Read the model definition and answer for the solid it produces. Units are mm, in the model's axes. Face numbers are marked on the shaded views. A direction names the side the tool comes from. Give positions to 0.01 mm unless a question says otherwise; leave off trailing zeros. Order: outer loops, then holes, each group sorted by start corner. A loop starts at its lowest first (then second) coordinate and runs counter-clockwise, first axis right, second up. Notation, with made-up numbers: (32, 0.5) -> (41, 0.5) arc R7 cw to (41, 9.5) -> close; hole circle Ø9 at (-20.75, 45.5). An arc over 180 degrees is marked (long way). Use one line per item in the form item = value.
```python
from build123d import *

# Parameters (mm, degrees)
F0_W     = 28
F0_H     = 30
F0_W_2   = 20
F0_H_2   = 22
F1_DEPTH = 10
F2_DEPTH = 15
F3_W     = 10
F3_H     = 10
F4_DEPTH = 5


with BuildPart() as f1:
    # F0 (on Top) → F1 (new body)
    with BuildSketch(Plane.XY):
        Rectangle(F0_W, F0_H)
        Rectangle(F0_W_2, F0_H_2, mode=Mode.SUBTRACT)
    extrude(amount=F1_DEPTH)

    # F0 (on Top) → F2 (join)
    with BuildSketch(Plane.XY):
        Rectangle(F0_W_2, F0_H_2)
    extrude(amount=F2_DEPTH)

    # F3 (on face) → F4 (join)
    with BuildSketch(Plane.XY.offset(15)):
        Rectangle(F3_W, F3_H)
    extrude(amount=F4_DEPTH)


solid = f1.part
```
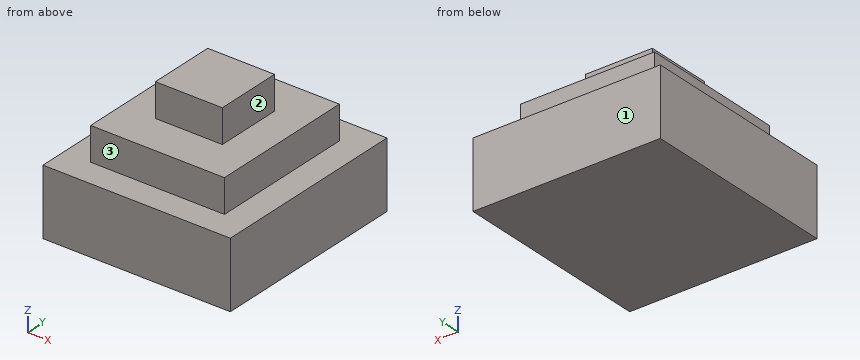
Item 1: The part is cut by section C-C on z = 10.5. Give the vertices of the cut face in (x, y).
Checks:
outline = (-10, -11) -> (10, -11) -> (10, 11) -> (-10, 11) -> close
Item 2: The part is cut by section D-D on x = 2.75. Give the vertices of the cut face in (y, z).
Checks:
outline = (-15, 0) -> (15, 0) -> (15, 10) -> (11, 10) -> (11, 15) -> (5, 15) -> (5, 20) -> (-5, 20) -> (-5, 15) -> (-11, 15) -> (-11, 10) -> (-15, 10) -> close
Item 3: The part is cut by section A-A on y = 5.5. Give the vertices of the cut face in (x, z), and give its area (3 significant figures).
Checks:
outline = (-14, 0) -> (14, 0) -> (14, 10) -> (10, 10) -> (10, 15) -> (-10, 15) -> (-10, 10) -> (-14, 10) -> close
area = 380 mm²
Item 4: The part is cut by section B-B on x = -7. Give the vertices of the cut face in (y, z), and give its area (3 significant figures).
Checks:
outline = (-15, 0) -> (15, 0) -> (15, 10) -> (11, 10) -> (11, 15) -> (-11, 15) -> (-11, 10) -> (-15, 10) -> close
area = 410 mm²
Item 5: Given pin 1 Ø1.5 at (x, y) = (4.5, -10) entering from +Z; pin 2 Ø2.5 at (y, z) = (-2.5, 11.5) entering from -X; pin 3 Ø2.5 at (y, z) = (-2, 18) entering from -X, each flat-ended and moving along its own axis, determine where each tip first touches the part or whether it passes through.
Checks:
pin_1 = 15
pin_2 = -10
pin_3 = -5
Item 6: Straight lines are drawn through the part: L1, parallel to Y at x = -8.25, z = 13.75; L2, parallel to Z at x = -2, y = 10.25; L3, parallel to X at y = 1.5, z = 14.5. For each, find the intervals that lie inside material, in ascending order. Write a range as from..to.
Checks:
L1 = -11..11
L2 = 0..15
L3 = -10..10
Item 7: Which of the six approach directions +Z, -Z, +X, -X, +Y, -Y give full straight-line access (tool end or side, diameter ignored) to the marked faces 1, 2 and 3?
Checks:
face_1 = +Z, -Z, +X, -X, +Y
face_2 = +Z, +X, +Y, -Y
face_3 = +Z, +X, -X, -Y
